Part model, mm, in its own coordinate system. Face numbers are marked on the shaded views. Round coordinates to 2 decimals unless told otherwise and drop trailing zeros. Write each loop counter-clockwise with the first axis right and the second up, starting at its lowest first coordinate (ties: lowest second). Pieces come first, ordered by that corner, then holes. Notation, with made-up numbers: (68.25, -12) -> (78.25, -12) arc R12 ccw to (78.25, 11) -> close; hole circle Ø2 at (-9.75, 34). An arc over 180 degrees is marked (long way). Return JSON: item names as keys, results as strings. Group by question number.
(1) Drop flat-ended pins along their axis: pin 1 Ø0.8 at (x, y) = (251, 1) entering from -Z (3 decimals); pin 2 Ø17 at (x, z) = (294.28, 152.4) entering from +Y. Give the stop position or say it passes through.
(2) Saw through at A-A (z = 275.5). List the corners of the cut face in (x, y) (3 decimals), plus the area to 3 significant figures.
(3) Drill centre lines: L1, parallel to Z at x = -190.5, y = 2.35 (3 decimals); L2, parallel to X at y = 0.4, z = 155 (3 decimals); L3, parallel to X at y = 0.1, z = -232 (3 decimals). Where is each one in solid material? Low to high. Write a range as from..to.
(4) Saw through at C-C (y = 1.9). State how many separate pieces and enclosed holes the cut face has, plus the area to 3 significant figures.
(5) Saw through at B-B (x = 248). List the corners of the cut face in (y, z) (3 decimals), plus the area to 3 significant figures.
(6) Mould opens along Y. For the marked faces 1 and 2 say: +Y half, -Y half, draft (parallel to the pull), parting line (faces both ways), or undercut.
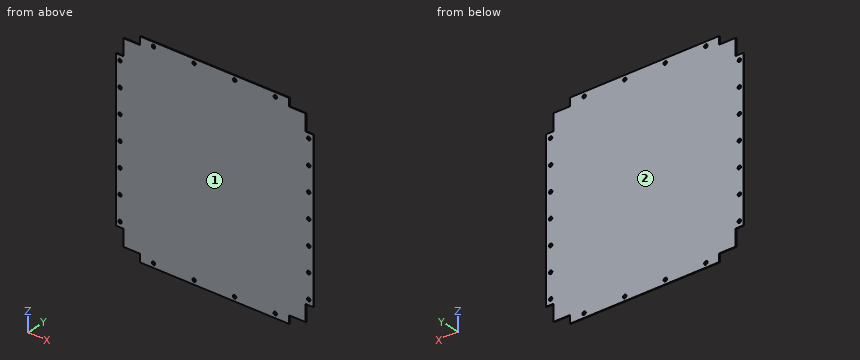
from build123d import *

# Parameters (mm, degrees)
SKETCH1_W           = 618.81
SKETCH1_H           = 642.21
BOSS_EXTRUDE1_DEPTH = 2.5
CUT_EXTRUDE1_DEPTH  = 2.5
SKETCH3_R           = 5.334
CUT_EXTRUDE2_DEPTH  = 10
SKETCH4_R           = 5.334
CUT_EXTRUDE3_DEPTH  = 10


with BuildPart() as part:
    # Sketch1 → Boss-Extrude1 (new body)
    with BuildSketch(Plane(origin=(0, 0, 0), x_dir=(1, 0, 0), z_dir=(0, 1, 0))):
        Rectangle(SKETCH1_W, SKETCH1_H)
    extrude(amount=BOSS_EXTRUDE1_DEPTH)

    # Sketch2 → Cut-Extrude1 (cut)
    with BuildSketch(Plane(origin=(0, 2.5, 0), x_dir=(1, 0, 0), z_dir=(0, 1, 0))):
        Polygon((-309.405, 321.105), (-233.205, 321.105), (-233.205, 296.445), (-284.745, 296.445), (-284.745, 244.905), (-309.405, 244.905), align=None)
        Polygon((-284.745, -244.905), (-309.405, -244.905), (-309.405, -321.105), (-233.205, -321.105), (-233.205, -296.445), (-284.745, -296.445), align=None)
        Polygon((284.745, -296.445), (284.745, -244.905), (309.405, -244.905), (309.405, -321.105), (233.205, -321.105), (233.205, -296.445), align=None)
        Polygon((284.745, 244.905), (309.405, 244.905), (309.405, 321.105), (233.205, 321.105), (233.205, 296.445), (284.745, 296.445), align=None)
    extrude(amount=-CUT_EXTRUDE1_DEPTH, mode=Mode.SUBTRACT)

    # Sketch3 → Cut-Extrude2 (cut)
    with BuildSketch(Plane(origin=(0, 0, 0), x_dir=(-1, 0, 0), z_dir=(0, -1, 0))):
        with Locations((-294.2768, -228.6018)):
            Circle(SKETCH3_R)
        with Locations((-294.2768, -152.4018)):
            Circle(SKETCH3_R)
        with Locations((-294.2768, -76.2018)):
            Circle(SKETCH3_R)
        with Locations((-294.2768, -0.0018)):
            Circle(SKETCH3_R)
        with Locations((-294.2768, 76.1982)):
            Circle(SKETCH3_R)
        with Locations((-294.2768, 152.3982)):
            Circle(SKETCH3_R)
        with Locations((-294.2768, 228.5982)):
            Circle(SKETCH3_R)
        with Locations((296.2732, -228.6018)):
            Circle(SKETCH3_R)
        with Locations((296.2732, -152.4018)):
            Circle(SKETCH3_R)
        with Locations((296.2732, -76.2018)):
            Circle(SKETCH3_R)
        with Locations((296.2732, -0.0018)):
            Circle(SKETCH3_R)
        with Locations((296.2732, 76.1982)):
            Circle(SKETCH3_R)
        with Locations((296.2732, 152.3982)):
            Circle(SKETCH3_R)
        with Locations((296.2732, 228.5982)):
            Circle(SKETCH3_R)
    extrude(amount=-CUT_EXTRUDE2_DEPTH, mode=Mode.SUBTRACT)

    # Sketch4 → Cut-Extrude3 (cut)
    with BuildSketch(Plane.XZ):
        with Locations((189.5018, 307.9768)):
            Circle(SKETCH4_R)
        with Locations((62.5018, 307.9768)):
            Circle(SKETCH4_R)
        with Locations((-64.4982, 307.9768)):
            Circle(SKETCH4_R)
        with Locations((-191.4982, 307.9768)):
            Circle(SKETCH4_R)
        with Locations((-191.4982, -307.9768)):
            Circle(SKETCH4_R)
        with Locations((-64.4982, -307.9768)):
            Circle(SKETCH4_R)
        with Locations((62.5018, -307.9768)):
            Circle(SKETCH4_R)
        with Locations((189.5018, -307.9768)):
            Circle(SKETCH4_R)
    extrude(amount=-CUT_EXTRUDE3_DEPTH, mode=Mode.SUBTRACT)


solid = part.part
Computed values:
{
 "1": {"pin 1": "z = -296.445", "pin 2": "y = 2.5"},
 "2": {"outline": "(-284.745, 0) -> (284.745, 0) -> (284.745, 2.5) -> (-284.745, 2.5) -> close", "area": "1,420 mm2"},
 "3": {"L1": "-321.105..-313.217, -302.737..302.737, 313.217..321.105", "L2": "-309.405..-300.932, -291.615..289.618, 298.935..309.405", "L3": "-309.405..-300.382, -292.165..290.168, 298.385..309.405"},
 "4": {"separate pieces": "1", "enclosed holes": "22", "area": "383,000 mm2"},
 "5": {"outline": "(0, -296.445) -> (2.5, -296.445) -> (2.5, 296.445) -> (0, 296.445) -> close", "area": "1,480 mm2"},
 "6": {"face 1": "-Y half", "face 2": "+Y half"}
}
